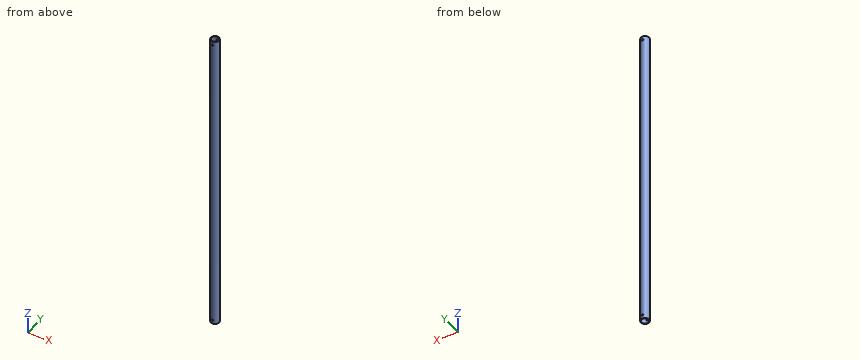
```python
from build123d import *

# Parameters (mm, degrees)
SKETCH1_R           = 6.35
SKETCH1_R_2         = 5.461
BOSS_EXTRUDE1_DEPTH = 242
SKETCH2_R           = 1.25
CUT_EXTRUDE1_DEPTH  = 7.35


with BuildPart() as part:
    # Sketch1 → Boss-Extrude1 (new body, symmetric)
    with BuildSketch(Plane.XY):
        Circle(SKETCH1_R)
        Circle(SKETCH1_R_2, mode=Mode.SUBTRACT)
    extrude(amount=BOSS_EXTRUDE1_DEPTH, both=True)

    # Sketch2 → Cut-Extrude1 (cut, symmetric)
    with BuildSketch(Plane(origin=(0, 0, 0), x_dir=(1, 0, 0), z_dir=(0, 1, 0))):
        with Locations((0, 236)):
            Circle(SKETCH2_R)
    cut_extrude1 = extrude(amount=CUT_EXTRUDE1_DEPTH, both=True, mode=Mode.SUBTRACT)

    # Mirror1: Cut-Extrude1 across plane
    add(cut_extrude1.mirror(Plane.XY), mode=Mode.SUBTRACT)


solid = part.part
```
Geometry check sheet. Reference: the model listing, model coordinates, mm. Coordinates: 2 decimals unless noted, no trailing zeros. Order: outer loops, then holes, each group sorted by start corner. A loop starts at its lowest first (then second) coordinate and runs counter-clockwise, first axis right, second up.
Q1. Depth check by flat-ended pin: pin 1 Ø1.5 at (y, z) = (2.5, 15.5) entering from -X; pin 2 Ø3 at (x, z) = (-4, -169.5) entering from +Y; pin 3 Ø1 at (y, z) = (3.5, 23) entering from +X. Enter the tip coordinate at first touch or a pass-through.
Reply:
pin 1: stops at x = -6.1
pin 2: stops at y = 5.84
pin 3: stops at x = 5.6
Q2. Sectioned sample at B-B on z = 58. Record the cut outline in (x, y).
Reply:
outline: circle Ø12.7 at (0, 0); hole circle Ø10.92 at (0, 0)
Q3. Sectioned sample at A-A on y = 0. Record the cut outline in (x, z).
Reply:
outline: (-6.35, -242) - (-5.46, -242) - (-5.46, 242) - (-6.35, 242) - close; (5.46, -242) - (6.35, -242) - (6.35, 242) - (5.46, 242) - close
Q4. Thickness scan on probe 1 along Z at (x, y) = (0, 6); probe 2 along Y at (x, z) = (0, -48); probe 3 along X at (y, z) = (1, -28.5). Record the ranges inside material, lowest first.
Reply:
probe 1: z = -242 to -237.25, -234.75 to 234.75, 237.25 to 242
probe 2: y = -6.35 to -5.46, 5.46 to 6.35
probe 3: x = -6.27 to -5.37, 5.37 to 6.27
